Part model, mm, in its own coordinate system. Face numbers are marked on the shaded views. A direction names the side the tool comes from. Give positions to 0.01 mm unless a question says otherwise; leave off trailing zeros. Loops run counter-clockwise (first coordinate to the right, second up) from the corner with the lowest first, then second, coordinate; pieces in that order, holes last. Notation, with made-up numbers: (4.25, 31) -> (55.25, 31) arc R38 ccw to (55.25, 70) -> close; hole circle Ø8 at (17.25, 22). An arc over 180 degrees is marked (long way). Write item = value, one per line.
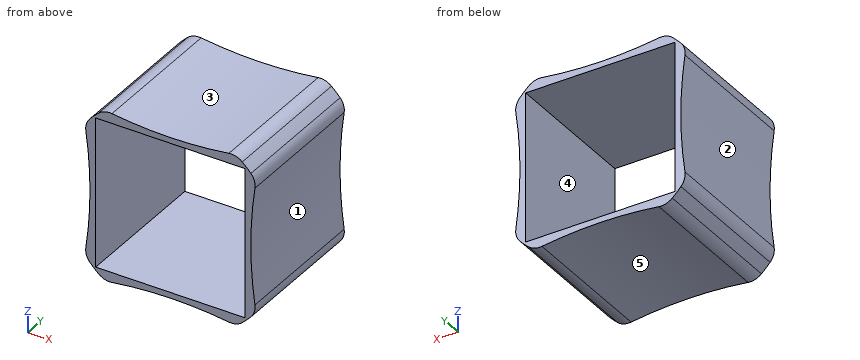
from build123d import *

# Parameters (mm, degrees)
F0_W     = 114.3
F0_H     = 114.3
F1_DEPTH = 107.95
F2_R     = 12.7


with BuildPart() as f1:
    # F0 (on Front) → F1 (new body)
    with BuildSketch(Plane.XZ):
        with BuildLine():
            ThreePointArc((50.235812, 65.5047), (0, 61.526428), (-50.235812, 65.5047))
            ThreePointArc((-50.235812, 65.5047), (-58.371665, 58.371665), (-65.5047, 50.235812))
            ThreePointArc((-65.5047, 50.235812), (-61.526428, 0), (-65.5047, -50.235812))
            ThreePointArc((-65.5047, -50.235812), (-58.371665, -58.371665), (-50.235812, -65.5047))
            ThreePointArc((-50.235812, -65.5047), (0, -61.526428), (50.235812, -65.5047))
            ThreePointArc((50.235812, -65.5047), (58.371665, -58.371665), (65.5047, -50.235812))
            ThreePointArc((65.5047, -50.235812), (61.526428, 0), (65.5047, 50.235812))
            ThreePointArc((65.5047, 50.235812), (58.371665, 58.371665), (50.235812, 65.5047))
        make_face()
        Rectangle(F0_W, F0_H, mode=Mode.SUBTRACT)
    extrude(amount=F1_DEPTH)

    # F2
    f2_edges = [f1.edges().sort_by_distance(p)[0] for p in [
        (-65.5047, -53.975, 50.235812),
        (-50.235812, -53.975, 65.5047),
        (50.235812, -53.975, 65.5047),
        (65.5047, -53.975, 50.235812),
        (50.235812, -53.975, -65.5047),
        (65.5047, -53.975, -50.235812),
        (-50.235812, -53.975, -65.5047),
        (-65.5047, -53.975, -50.235812),
    ]]
    fillet(f2_edges, radius=F2_R)


solid = f1.part
1) Drop flat-ended pins along their axis: P1, Ø3, axis at y = -37, z = 2.5, coming from the -X side; P2, Ø1, axis at y = -46, z = 37, coming from the +X side; P3, Ø6, axis at y = -63, z = 50, coming from the +X side. Give the stop position or say it passes through.
Resolved:
P1 = -61.55
P2 = 63.74
P3 = 64.79
2) Drill centre lines: line 1 along X through (y, z) = (-30.5, 47.5); line 2 along X through (y, z) = (-39.5, 7); line 3 along Z through (x, y) = (-0.5, -99.5). Where is each one in solid material? Low to high. Write a range as [from, to].
Resolved:
line_1 = [-64.77, -57.15], [57.15, 64.77]
line_2 = [-61.6, -57.15], [57.15, 61.6]
line_3 = [-61.53, -57.15], [57.15, 61.53]
3) Pull direction X, two halves, no side cores. Call the marked faces 1, 2 and 3: pulls with the +X half, pulls with the -X half, needs draft (parallel to the pull), parting line crosses it, or undercut.
Resolved:
face_1 = pulls with the +X half
face_2 = pulls with the -X half
face_3 = undercut
4) Slice it at A-A, the plane z = 35.5. List the corners of the cut face in (x, y).
Resolved:
outline = (-63.51, -107.95) -> (-57.15, -107.95) -> (-57.15, 0) -> (-63.51, 0) -> close; (57.15, -107.95) -> (63.51, -107.95) -> (63.51, 0) -> (57.15, 0) -> close
5) Slice it at B-B, the plane x = -24.5. List the corners of the cut face in (y, z), and give its area (3 significant figures).
Resolved:
outline = (-107.95, -62.47) -> (0, -62.47) -> (0, -57.15) -> (-107.95, -57.15) -> close; (-107.95, 57.15) -> (0, 57.15) -> (0, 62.47) -> (-107.95, 62.47) -> close
area = 1,150 mm²
6) Which spindle directions (+Z, -Z, +X, -X, +Y, -Y) get a long thin tool onto all of the face, cutting with end or side? Do the marked faces 4 and 5. Say none if no direction does.
Resolved:
face_4 = +Y, -Y
face_5 = -Z, +Y, -Y
